Job drawing, mm, ordinate dimensions from the low corner. One solid piece. A direction names the side the tool comes from. Round coordinates to 2 decimals unless told otherwise and drop trailing zeros. Order: outer loops, then holes, each group sorted by start corner. A loop starts at its lowest first (then second) coordinate and runs counter-clockwise, first axis right, second up. Notation, with made-up numbers: (2.5, 88.5) -> (32.5, 88.5) arc R21 cw to (32.5, 92.5) -> close; hole circle Ø4 at (53.5, 61). An arc over 180 degrees is marked (long way). Use CSV: the item, a comma, the result in double quotes.
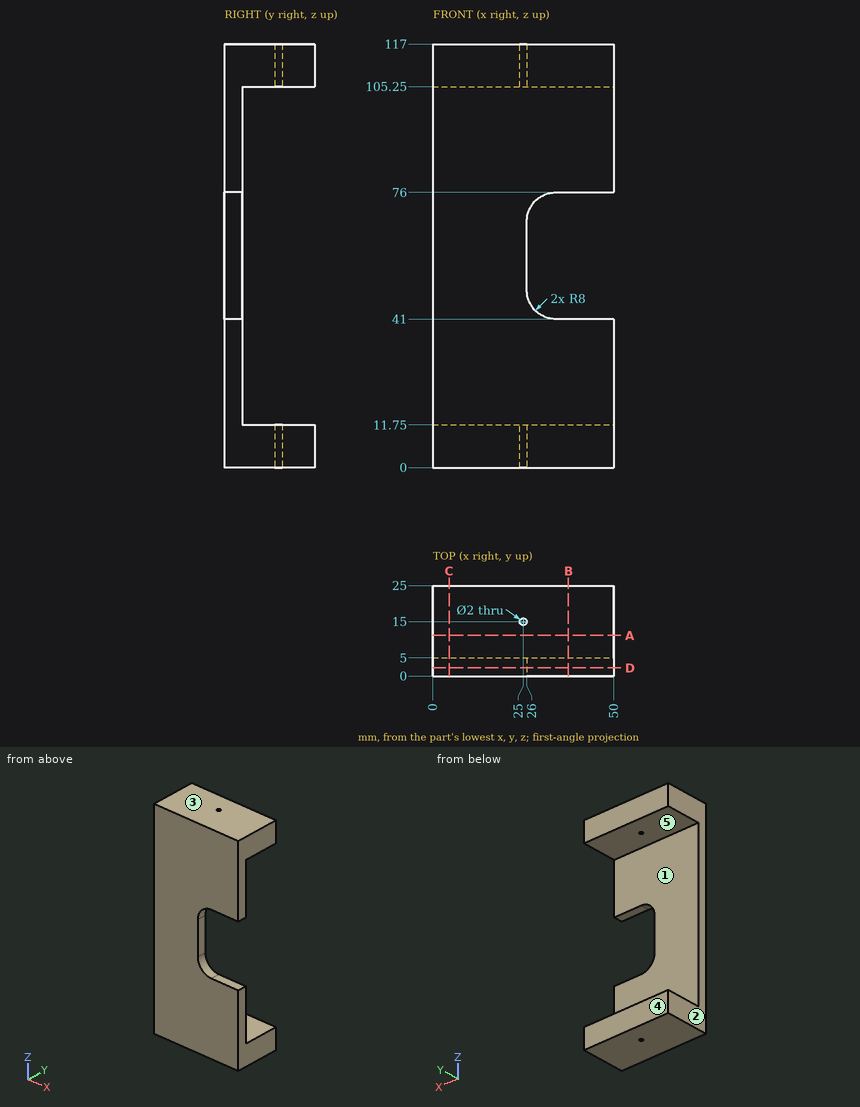
(1) Probe probe 1 along Y at (x, z) = (25, 7); probe 2 along Z at (x, y) = (30.5, 15.5); probe 3 along Y at (x, z) = (10.5, 30). List the from-to ranges inside material, lowest first. Write a range as [from, to].
Reply:
probe 1,"[0, 14], [16, 25]"
probe 2,"[0, 11.75], [105.25, 117]"
probe 3,"[0, 5]"
(2) Pull direction Z, two halves, no side cores. Call the marked faces 3, 4 and 5: released by +Z, released by -Z, zero draft, split by the parting line, or undercut.
Reply:
face 3,"released by +Z"
face 4,"zero draft"
face 5,"undercut"
(3) Drop flat-ended pins along their axis: P1, Ø3, axis at x = 8, z = 72, coming from the +Y side; P2, Ø5.5, axis at y = 3, z = 59.5, coming from the +X side. Give the stop position or say it passes through.
Reply:
P1,"y = 5"
P2,"x = 26"
(4) Cut at A-A, the plane y = 11.25. Give the cut face in (x, z), then the cut area to 4 significant figures.
Reply:
outline,"(0, 0) -> (50, 0) -> (50, 11.75) -> (0, 11.75) -> close; (0, 105.25) -> (50, 105.25) -> (50, 117) -> (0, 117) -> close"
area,"1,175 mm2"
(5) Cut at C-C, the plane x = 4.5. Give the cut face in (y, z), then the cut area to 4 significant figures.
Reply:
outline,"(0, 0) -> (25, 0) -> (25, 11.75) -> (5, 11.75) -> (5, 105.25) -> (25, 105.25) -> (25, 117) -> (0, 117) -> close"
area,"1,055 mm2"
(6) Cut at D-D, the plane y = 2.25. Give the cut face in (x, z).
Reply:
outline,"(0, 0) -> (50, 0) -> (50, 41) -> (34, 41) arc R8 cw to (26, 49) -> (26, 68) arc R8 cw to (34, 76) -> (50, 76) -> (50, 117) -> (0, 117) -> close"
(7) Cut at B-B, the plane x = 37.5. Give the cut face in (y, z).
Reply:
outline,"(0, 0) -> (25, 0) -> (25, 11.75) -> (5, 11.75) -> (5, 41) -> (0, 41) -> close; (0, 76) -> (5, 76) -> (5, 105.25) -> (25, 105.25) -> (25, 117) -> (0, 117) -> close"
(8) Which spindle directions (+Z, -Z, +X, -X, +Y, -Y) get a long thin tool onto all of the face, cutting with end or side? Do the marked faces 1 and 2. Say none if no direction does.
Reply:
face 1,"+X, -X, +Y"
face 2,"+Z, -Z, -X, +Y, -Y"
